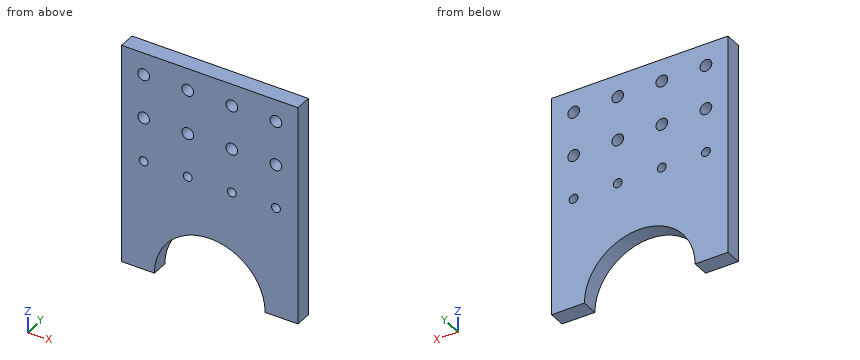
from build123d import *

# Parameters (mm, degrees)
SKETCH1_W                   = 101.6
SKETCH1_H                   = 127
BOSS_EXTRUDE1_DEPTH         = 9.525
SKETCH2_R                   = 31.877
CUT_EXTRUDE1_DEPTH          = 10.525
F_1_4_CLEARANCE_HOLE1_D     = 6.7564
LPATTERN1_COUNT             = 2
LPATTERN1_PITCH             = 25.4
LPATTERN1_COUNT_DIR2        = 4
LPATTERN1_PITCH_DIR2        = 25.4
TAP_DRILL_FOR_1_4_20_TAP1_D = 5.1054
LPATTERN2_COUNT             = 4
LPATTERN2_PITCH             = 25.4


with BuildPart() as part:
    # Sketch1 → Boss-Extrude1 (new body)
    with BuildSketch(Plane(origin=(0, 0, 0), x_dir=(1, 0, 0), z_dir=(0, 1, 0))):
        with Locations((50.8, 63.5)):
            Rectangle(SKETCH1_W, SKETCH1_H)
    extrude(amount=BOSS_EXTRUDE1_DEPTH)

    # Sketch2 → Cut-Extrude1 (cut, through all)
    with BuildSketch(Plane(origin=(0, 9.525, 0), x_dir=(1, 0, 0), z_dir=(0, 1, 0))):
        with Locations((50.8, 127)):
            Circle(SKETCH2_R)
    extrude(amount=-CUT_EXTRUDE1_DEPTH, mode=Mode.SUBTRACT)

    # 1/4 Clearance Hole1 (through all)
    with Locations(Plane(origin=(0, 9.525, 0), x_dir=(-1, 0, 0), z_dir=(0, 1, 0))):
        with Locations((-12.7, -12.7)):
            f_1_4_clearance_hole1 = Hole(F_1_4_CLEARANCE_HOLE1_D / 2)

    # LPattern1: 1_4 Clearance Hole1 2 × 4
    with Locations(*[(j * LPATTERN1_PITCH_DIR2, 0, -i * LPATTERN1_PITCH) for i in range(LPATTERN1_COUNT) for j in range(LPATTERN1_COUNT_DIR2) if (i, j) != (0, 0)]):
        add(f_1_4_clearance_hole1, mode=Mode.SUBTRACT)

    # Tap Drill for 1/4-20 Tap1 (through all)
    with Locations(Plane(origin=(0, 9.525, 0), x_dir=(-1, 0, 0), z_dir=(0, 1, 0))):
        with Locations((-12.7, -63.5)):
            tap_drill_for_1_4_20_tap1 = Hole(TAP_DRILL_FOR_1_4_20_TAP1_D / 2)

    # LPattern2: Tap Drill for 1/4-20 Tap1 ×4
    with Locations(*[(i * LPATTERN2_PITCH, 0, 0) for i in range(1, LPATTERN2_COUNT)]):
        add(tap_drill_for_1_4_20_tap1, mode=Mode.SUBTRACT)


solid = part.part
For this review, take the finished solid that the model builds, in its own axes (mm). Round coordinates to 2 decimals unless told otherwise and drop trailing zeros. Order: outer loops, then holes, each group sorted by start corner. A loop starts at its lowest first (then second) coordinate and runs counter-clockwise, first axis right, second up. Notation, with made-up numbers: M -14,64 L 40,64 A22 ccw 40,70 Z; hole C 57.25,26 d1. An arc over 180 degrees is marked long. Use a Markdown table: item, result. Add a question column.
Item 1: Add section B-B, the plane z = -63.5. Give the boundary of the cut face in (x, y) (3 decimals), then the cut area to 3 significant figures.
Item 2: Add section A-A, the plane x = 12.7. Give the boundary of the cut face in (y, z) (3 decimals), then the cut area to 3 significant figures.
Item 3: Insertion check: pin 1 (5 mm diameter, centred on x = 63, y = 3, fed in from -Z). The pin has a flat end and moves straight along its axis. Give the tip position at first contact, or say it passes through.
Item 4: To check wall thickness, follow line 1 along Z through (x, y) = (88.9, 4); line 2 along X through (y, z) = (4.5, -13); line 3 along Z through (x, y) = (63.5, 4.5). State the ranges of each line that lie inside material, in increasing order.
Item 5: Add section C-C, the plane y = 4.5. State how many separate pieces and enclosed holes the cut face has, then the cut area to 3 significant figures.
Item 6: Add section D-D, the plane z = -12.7. Give the boundary of the cut face in (x, y) (3 decimals).
Geometry results:
| question | item | result |
|---|---|---|
| 1 | outline | M 0,0 L 10.147,0 L 10.147,9.525 L 0,9.525 Z; M 15.253,0 L 35.547,0 L 35.547,9.525 L 15.253,9.525 Z; M 40.653,0 L 60.947,0 L 60.947,9.525 L 40.653,9.525 Z; M 66.053,0 L 86.347,0 L 86.347,9.525 L 66.053,9.525 Z; M 91.453,0 L 101.6,0 L 101.6,9.525 L 91.453,9.525 Z |
| 1 | area | 773 mm² |
| 2 | outline | M 0,-127 L 9.525,-127 L 9.525,-66.053 L 0,-66.053 Z; M 0,-60.947 L 9.525,-60.947 L 9.525,-41.478 L 0,-41.478 Z; M 0,-34.722 L 9.525,-34.722 L 9.525,-16.078 L 0,-16.078 Z; M 0,-9.322 L 9.525,-9.322 L 9.525,0 L 0,0 Z |
| 2 | area | 1,030 mm² |
| 3 | pin 1 | stops at z = -98.71 |
| 4 | line 1 | z = -127 to -66.05, -60.95 to -41.48, -34.72 to -16.08, -9.32 to 0 |
| 4 | line 2 | x = 0 to 9.34, 16.06 to 34.74, 41.46 to 60.14, 66.86 to 85.54, 92.26 to 101.6 |
| 4 | line 3 | z = -97.76 to -66.05, -60.95 to -41.48, -34.72 to -16.08, -9.32 to 0 |
| 5 | separate pieces | 1 |
| 5 | enclosed holes | 12 |
| 5 | area | 10,900 mm² |
| 6 | outline | M 0,0 L 9.322,0 L 9.322,9.525 L 0,9.525 Z; M 16.078,0 L 34.722,0 L 34.722,9.525 L 16.078,9.525 Z; M 41.478,0 L 60.122,0 L 60.122,9.525 L 41.478,9.525 Z; M 66.878,0 L 85.522,0 L 85.522,9.525 L 66.878,9.525 Z; M 92.278,0 L 101.6,0 L 101.6,9.525 L 92.278,9.525 Z |
